Part model, mm, in its own coordinate system. Face numbers are marked on the shaded views. A direction names the side the tool comes from. Coordinates: 2 decimals unless noted, no trailing zeros. Order: outer loops, then holes, each group sorted by start corner. A loop starts at its lowest first (then second) coordinate and runs counter-clockwise, first axis right, second up. Notation, with made-up numbers: (-12, -25) - (21, -25) arc R24 ccw to (21, 4) - close; hole circle Ø3 at (79, -10.5). An arc over 180 degrees is marked (long way). Use a Markdown table: item, result. Add a question column.
1) Saw through at B-B on x = -19.5. List the corners of the cut face in (y, z), then the cut area to 3 significant figures.
2) Two-plate mould, pull along Y, no slides. Class the marked faces 1, 2 and 3: +Y half, -Y half, draft (parallel to the pull), parting line (faces both ways), or undercut.
3) Saw through at A-A on y = -10.5. List the corners of the cut face in (x, z) (3 decimals).
4) Drop a flat-ended pin along its axis: P1, Ø4.5, axis at y = 12, z = 5, coming from the -X side. Give the stop position or say it passes through.
5) Wall check: L1, parallel to Z at x = 24.5, y = -11.5; L2, parallel to Y at x = -16.5, z = 7; L3, parallel to Z at x = 2.5, y = -9 (3 decimals). Give the ranges that are in metal, low to high. Write a range as [from, to].
6) Tool access for the marked faces 4 and 5: list every direction of +Z, -Z, +X, -X, +Y, -Y with a clear straight run to the whole face (end or side of a thin tool).
7) Saw through at D-D on y = 23. List the corners of the cut face in (x, z).
8) Saw through at C-C on z = 19. List the corners of the cut face in (x, y), then the cut area to 3 significant figures.
```python
from build123d import *

# Parameters (mm, degrees)
F0_W      = 91.44
F0_H      = 63.5
F1_DEPTH  = 25.4
F3_W      = 62.104847
F3_H      = 24.073936
F4_DEPTH  = 89.154
F5_W      = 91.44
F5_H      = 0.576332
F6_DEPTH  = 63.2206
F7_W      = 11.196822
F7_H      = 30.827232
F8_DEPTH  = 15.24
F9_W      = 11.196822
F9_H      = 30.827232
F10_DEPTH = 0.635


with BuildPart() as f1:
    # F0 (on Top) → F1 (new body)
    with BuildSketch(Plane.XY):
        Rectangle(F0_W, F0_H)
    extrude(amount=F1_DEPTH)

    # F3 (on face) → F4 (cut)
    with BuildSketch(Plane(origin=(-45.72, 0, 0), x_dir=(0, -1, 0), z_dir=(-1, 0, 0))):
        with Locations((0.017024, 12.710826)):
            Rectangle(F3_W, F3_H)
    extrude(amount=-F4_DEPTH, mode=Mode.SUBTRACT)

    # F5 (on face) → F6 (join)
    with BuildSketch(Plane.XZ.offset(31.75)):
        with Locations((0, 16.477615)):
            Rectangle(F5_W, F5_H)
    extrude(amount=-F6_DEPTH)

    # F7 (on face) → F8 (cut)
    with BuildSketch(Plane.XY.offset(25.4)):
        Rectangle(F7_W, F7_H)
    extrude(amount=-F8_DEPTH, mode=Mode.SUBTRACT)

    # F9 (on face) → F10 (join)
    with BuildSketch(Plane.XY.offset(25.4)):
        Rectangle(F9_W, F9_H)
    extrude(amount=-F10_DEPTH)


solid = f1.part
```
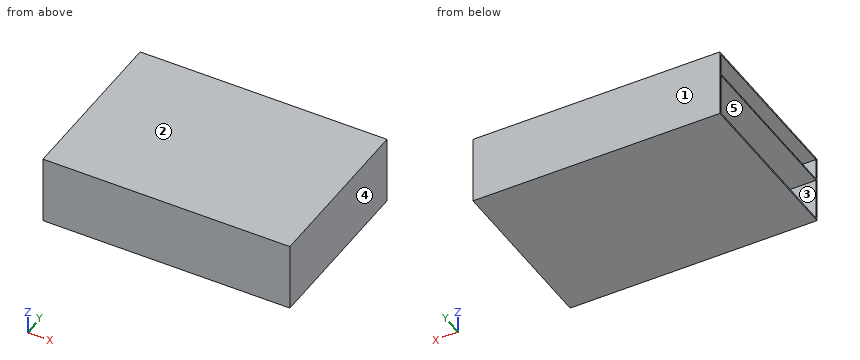
Results are:
| question | item | result |
|---|---|---|
| 1 | outline | (-31.75, 0) - (31.75, 0) - (31.75, 25.4) - (-31.75, 25.4) - close; hole (-31.07, 0.67) - (31.04, 0.67) - (31.04, 16.19) - (-31.07, 16.19) - close; hole (-31.07, 16.77) - (31.04, 16.77) - (31.04, 24.75) - (-31.07, 24.75) - close |
| 1 | area | 154 mm2 |
| 2 | face 1 | +Y half |
| 2 | face 2 | draft |
| 2 | face 3 | undercut |
| 3 | outline | (-45.72, 0) - (45.72, 0) - (45.72, 25.4) - (-45.72, 25.4) - (-45.72, 24.748) - (-5.598, 24.748) - (-5.598, 24.765) - (5.598, 24.765) - (5.598, 24.748) - (43.434, 24.748) - (43.434, 16.766) - (5.598, 16.766) - (5.598, 16.189) - (43.434, 16.189) - (43.434, 0.674) - (-45.72, 0.674) - close; (-45.72, 16.189) - (-5.598, 16.189) - (-5.598, 16.766) - (-45.72, 16.766) - close |
| 4 | P1 | x = 43.43 |
| 5 | L1 | [0, 0.67], [16.19, 16.77], [24.75, 25.4] |
| 5 | L2 | [-31.75, -31.07], [31.04, 31.75] |
| 5 | L3 | [0, 0.674], [24.765, 25.4] |
| 6 | face 4 | +Z, -Z, +X, +Y, -Y |
| 6 | face 5 | -X |
| 7 | outline | (-45.72, 0) - (45.72, 0) - (45.72, 25.4) - (-45.72, 25.4) - (-45.72, 24.75) - (43.43, 24.75) - (43.43, 16.77) - (-45.72, 16.77) - (-45.72, 16.19) - (43.43, 16.19) - (43.43, 0.67) - (-45.72, 0.67) - close |
| 8 | outline | (-45.72, -31.75) - (45.72, -31.75) - (45.72, 31.75) - (-45.72, 31.75) - (-45.72, 31.04) - (43.43, 31.04) - (43.43, -31.07) - (-45.72, -31.07) - close |
| 8 | area | 270 mm2 |
